Design review of the part built by this model. Coordinates are the model's own, in mm. Face numbers are marked on the shaded views. A direction names the side the tool comes from. Coordinates: 2 decimals unless noted, no trailing zeros. Loops run counter-clockwise (first coordinate to the right, second up) from the corner with the lowest first, then second, coordinate; pieces in that order, holes last. Notation, with made-up numbers: (12.5, -14.5) -> (38.5, -14.5) arc R28 cw to (38.5, 20.5) -> close; hole circle Ø10 at (61.25, 33.25). An arc over 180 degrees is marked (long way). Answer in a Markdown table with one row per item.
```python
from build123d import *

# Parameters (mm, degrees)
BOX003_W     = 15
BOX003_H     = 15
BOX003_DEPTH = 3
BOX001_W     = 5.5
BOX001_H     = 5.5
BOX001_DEPTH = 6
BOX002_W     = 7.5
BOX002_H     = 7.5
BOX002_DEPTH = 6
FILLET_R     = 2.5
FILLET001_R  = 1


with BuildPart() as cube002:
    # Box003 → Box003 (new body)
    with BuildSketch(Plane.XY.offset(-2.5)):
        with Locations((7.5, 7.5)):
            Rectangle(BOX003_W, BOX003_H)
    extrude(amount=BOX003_DEPTH)


with BuildPart() as inf:
    # Box001 → Box001 (new body)
    with BuildSketch(Plane(origin=(1, 1, 1), x_dir=(1, 0, 0), z_dir=(0, 0, 1))):
        with Locations((2.75, 2.75)):
            Rectangle(BOX001_W, BOX001_H)
    extrude(amount=BOX001_DEPTH)


with BuildPart() as fillet001:
    # Box002 → Box002 (new body)
    with BuildSketch(Plane.XY):
        with Locations((3.75, 3.75)):
            Rectangle(BOX002_W, BOX002_H)
    extrude(amount=BOX002_DEPTH)

    # Cut001: cut inf
    add(inf.part, mode=Mode.SUBTRACT)


with BuildPart() as fillet001_1:
    # Cut001 placement: moved
    add(fillet001.part.moved(Location((3.75, 3.75, 0))))

    # Fusion: union Cube002
    add(cube002.part)

    # Fillet
    fillet_edges = [fillet001_1.edges().sort_by_distance(p)[0] for p in [
        (3.75, 7.5, 0.5),
        (7.5, 3.75, 0.5),
        (11.25, 7.5, 0.5),
        (7.5, 11.25, 0.5),
    ]]
    fillet(fillet_edges, radius=FILLET_R)

    # Fillet001
    fillet001_edges = [fillet001_1.edges().sort_by_distance(p)[0] for p in [
        (0, 0, -1),
        (0, 15, -1),
        (15, 15, -1),
        (15, 0, -1),
    ]]
    fillet(fillet001_edges, radius=FILLET001_R)


solid = fillet001_1.part
```
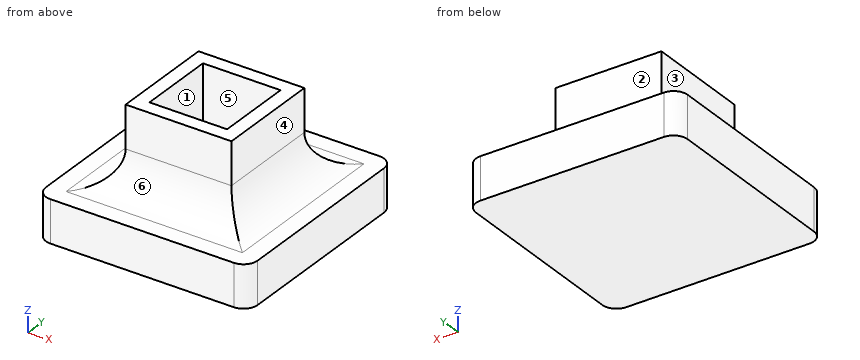
(1) Draft analysis for pull direction Y (two halves, no side actions). For the marked faces 4, 5 and 6, state which applies: pulls with the +Y half, pulls with the -Y half, needs draft (parallel to the pull), parting line crosses it, or undercut.
Evaluation:
| item | result |
|---|---|
| face 4 | needs draft |
| face 5 | undercut |
| face 6 | pulls with the -Y half |
(2) For pin 1 (3.5 mm diameter, centred on x = 6, z = 4.5, fed in from -Y); pin 2 (2.5 mm diameter, centred on y = 8, z = 2.5, fed in from +X); pin 3 (3.5 mm diameter, centred on y = 6.5, z = 5, fed in from -X); pin 4 (3 mm diameter, centred on x = 2, z = 4.5, fed in from -Y), all flat-tipped, find the tip position at first contact; note any pin that passes through.
Evaluation:
| item | result |
|---|---|
| pin 1 | stops at y = 3.74 |
| pin 2 | stops at x = 11.96 |
| pin 3 | stops at x = 3.75 |
| pin 4 | passes through |
(3) Take a section at B-B on y = 11. Give the boundary of the cut face in (x, z).
Evaluation:
| item | result |
|---|---|
| outline | (0, -2.5) -> (15, -2.5) -> (15, 0.5) -> (13.75, 0.5) arc R2.5 cw to (11.25, 3) -> (11.25, 6) -> (3.75, 6) -> (3.75, 3) arc R2.5 cw to (1.25, 0.5) -> (0, 0.5) -> close |
(4) To check wall thickness, follow probe 1 along Y at (x, z) = (9.25, 4.75); probe 2 along X at (y, z) = (10.75, 5.25). State the ranges of each line that lie inside material, in increasing order.
Evaluation:
| item | result |
|---|---|
| probe 1 | y = 3.75 to 4.75, 10.25 to 11.25 |
| probe 2 | x = 3.75 to 11.25 |
(5) Take a section at C-C on x = 3.25. Give the boundary of the cut face in (y, z), and give its area (3 significant figures).
Evaluation:
| item | result |
|---|---|
| outline | (0, -2.5) -> (15, -2.5) -> (15, 0.5) -> (13.75, 0.5) arc R2.5 cw to (11.75, 1.5) -> (3.25, 1.5) arc R2.5 cw to (1.25, 0.5) -> (0, 0.5) -> close |
| area | 54.7 mm² |
(6) Take a section at D-D on z = 1.5. Give the boundary of the cut face in (x, y), and give its area (3 significant figures).
Evaluation:
| item | result |
|---|---|
| outline | (3.25, 3.25) -> (11.75, 3.25) -> (11.75, 11.75) -> (3.25, 11.75) -> close; hole (4.75, 4.75) -> (10.25, 4.75) -> (10.25, 10.25) -> (4.75, 10.25) -> close |
| area | 42.0 mm² |
(7) Tool access review of the marked faces 1, 2 and 3: name each direction out of +Z, -Z, +X, -X, +Y, -Y from which nothing blocks a thin tool from reaching the whole face with its end or side.
Evaluation:
| item | result |
|---|---|
| face 1 | +Z |
| face 2 | +Z, +X, -X, +Y |
| face 3 | +Z, -X, +Y, -Y |
(8) Take a section at A-A on z = 3.5. Give the boundary of the cut face in (x, y).
Evaluation:
| item | result |
|---|---|
| outline | (3.75, 3.75) -> (11.25, 3.75) -> (11.25, 11.25) -> (3.75, 11.25) -> close; hole (4.75, 4.75) -> (10.25, 4.75) -> (10.25, 10.25) -> (4.75, 10.25) -> close |
